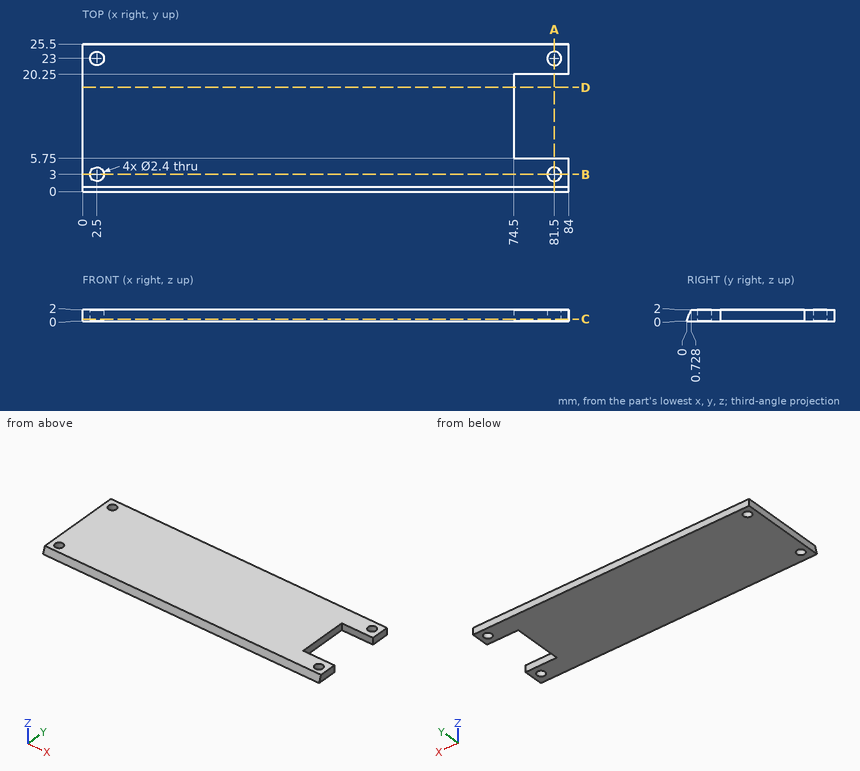
Geometry: see drawing. Coordinates: mm, zero at the bounding-box minimum. Give positions to 0.01 mm unless a question says otherwise; leave off trailing zeros. Write each loop counter-clockwise with the first axis right and the second up, starting at its lowest first coordinate (ties: lowest second). Pieces come first, ordered by that corner, then holes. Notation, with made-up numbers: (-27, -2.75) - (-10, -2.75) arc R10 cw to (-10, 15.25) - close; hole circle Ø5 at (41.25, 2). An arc over 180 degrees is marked (long way). Return JSON: item names as keys, results as strings. Group by question number.
1) First-contact query: P1, Ø1, axis at y = 10, z = 1, coming from the +X side; P2, Ø1, axis at x = 81.5, z = 1, coming from the -Y side. Flat tips, straight axial feed; report the tip coordinate or a pass-through.
2) Section C-C on z = 0.35. Return the cut outline in (x, y).
3) Section A-A on x = 81.5. Return the cut outline in (y, z).
4) Section D-D on y = 18. Return the cut outline in (x, z), plus the area to 3 significant figures.
5) Section B-B on y = 3. Return the cut outline in (x, z).
6) Line query: line 1 (Y direction, x = 81.5, z = 0.9); line 2 (Y direction, x = 81.5, z = 1.45); line 3 (Y direction, x = 2.5, z = 0.8). Output: solid intervals per line, ascending.
Filled in:
{
 "1": {"P1": "stops at x = 74.5", "P2": "stops at y = 0.18"},
 "2": {"outline": "(0, 0.13) - (84, 0.13) - (84, 5.75) - (74.5, 5.75) - (74.5, 20.25) - (84, 20.25) - (84, 25.5) - (0, 25.5) - close; hole circle Ø2.4 at (2.5, 3); hole circle Ø2.4 at (2.5, 23); hole circle Ø2.4 at (81.5, 3); hole circle Ø2.4 at (81.5, 23)"},
 "3": {"outline": "(0, 0) - (1.8, 0) - (1.8, 2) - (0.73, 2) - close; (4.2, 0) - (5.75, 0) - (5.75, 2) - (4.2, 2) - close; (20.25, 0) - (21.8, 0) - (21.8, 2) - (20.25, 2) - close; (24.2, 0) - (25.5, 0) - (25.5, 2) - (24.2, 2) - close"},
 "4": {"outline": "(0, 0) - (74.5, 0) - (74.5, 2) - (0, 2) - close", "area": "149 mm^2"},
 "5": {"outline": "(0, 0) - (1.3, 0) - (1.3, 2) - (0, 2) - close; (3.7, 0) - (80.3, 0) - (80.3, 2) - (3.7, 2) - close; (82.7, 0) - (84, 0) - (84, 2) - (82.7, 2) - close"},
 "6": {"line 1": "y = 0.33 to 1.8, 4.2 to 5.75, 20.25 to 21.8, 24.2 to 25.5", "line 2": "y = 0.53 to 1.8, 4.2 to 5.75, 20.25 to 21.8, 24.2 to 25.5", "line 3": "y = 0.29 to 1.8, 4.2 to 21.8, 24.2 to 25.5"}
}
